from build123d import *

# Parameters (mm, degrees)
F0_R      = 26.5
F1_DEPTH  = 200
F2_R      = 12.5
F3_DEPTH  = 30
F4_W      = 21.5
F4_H      = 60
F5_DEPTH  = 55
F8_DEPTH  = 10
F9_R      = 10
F10_DEPTH = 140


with BuildPart() as f1:
    # F0 (on Front) → F1 (new body)
    with BuildSketch(Plane.XZ):
        Circle(F0_R)
    extrude(amount=F1_DEPTH)

    # F2 (on Right) → F3 (cut, symmetric)
    with BuildSketch(Plane.YZ):
        with Locations((-20, 0)):
            Circle(F2_R)
    extrude(amount=F3_DEPTH, both=True, mode=Mode.SUBTRACT)

    # F4 (on Front) → F5 (cut)
    with BuildSketch(Plane.XZ):
        Rectangle(F4_W, F4_H)
    extrude(amount=F5_DEPTH, mode=Mode.SUBTRACT)

    # F7 (on offset) → F8 (cut)
    with BuildSketch(Plane.YZ.offset(22)):
        with BuildLine():
            Line((-42.6307463948, 4.9999999723), (-172.6307456746, 4.986315794))
            ThreePointArc((-172.6307456746, 4.986315794), (-177.630219249, -0.0147382518), (-172.6286375277, -5.0136839281))
            Line((-172.6286375277, -5.0136839281), (-42.6286382479, -4.9999997498))
            ThreePointArc((-42.6286382479, -4.9999997498), (-37.6302201914, 0.0010540735), (-42.6307463948, 4.9999999723))
        make_face()
    extrude(amount=F8_DEPTH, mode=Mode.SUBTRACT)

    # F9 (on face) → F10 (cut)
    with BuildSketch(Plane.XZ.offset(200)):
        Circle(F9_R)
    extrude(amount=-F10_DEPTH, mode=Mode.SUBTRACT)


solid = f1.part
Design review of the part built by this model. Coordinates are the model's own, in mm. A direction names the side the tool comes from. Give positions to 0.01 mm unless a question says otherwise; leave off trailing zeros. Loops run counter-clockwise (first coordinate to the right, second up) from the corner with the lowest first, then second, coordinate; pieces in that order, holes last. Notation, with made-up numbers: M 20.25,25 L 42.25,25 A15 ccw 42.25,36 Z; hole C -5.5,-23 d9. An arc over 180 degrees is marked long. Answer as a JSON object with one key per item and string values.
Item 1: Wall thickness on line 1 along Y through (x, z) = (14.5, 0); line 2 along Z through (x, y) = (0, -156); line 3 along X through (y, z) = (-151, -7.5): over which ranges is each line inside the solid? List them lowest first.
Output values:
{"line 1": "y = -200 to -32.5, -7.5 to 0", "line 2": "z = -26.5 to -10, 10 to 26.5", "line 3": "x = -25.42 to -6.61, 6.61 to 25.42"}
Item 2: We need section A-A (z = 7). State the section outline as (x, y) points.
Output values:
{"outline": "M -25.56,-200 L -7.14,-200 L -7.14,-60 L 7.14,-60 L 7.14,-200 L 25.56,-200 L 25.56,-30.36 L 10.75,-30.36 L 10.75,-55 L -10.75,-55 L -10.75,-30.36 L -25.56,-30.36 Z; M -25.56,-9.64 L -10.75,-9.64 L -10.75,0 L -25.56,0 Z; M 10.75,-9.64 L 25.56,-9.64 L 25.56,0 L 10.75,0 Z"}
Item 3: We need section C-C (y = -20). State the section outline as (x, z) points.
Output values:
{"outline": "M -23.37,-12.5 A26.5 ccw -10.75,-24.22 L -10.75,-12.5 Z; M -23.37,12.5 L -10.75,12.5 L -10.75,24.22 A26.5 ccw Z; M 10.75,-24.22 A26.5 ccw 23.37,-12.5 L 10.75,-12.5 Z; M 10.75,12.5 L 23.37,12.5 A26.5 ccw 10.75,24.22 Z"}
Item 4: Machinability: for faces 1 (the face through (-2.17, -130.98, -9.76)), 2 (the face through (10.75, -33, 0)), 3 (the face through (24.22, -177.63, 0.1)), 4 (the face through (11, -200, 0)), 5 (the face through (-18.515, -8.077, 3.755)), which of the approach directions +Z, -Z, +X, -X, +Y, -Y give a long, thin tool a straight path to every point of the face, cutting with its end or side? Answer none if there is none.
Output values:
{"face 1": "-Y", "face 2": "+Z, -Z, +Y", "face 3": "+X", "face 4": "+Z, -Z, +X, -X, -Y", "face 5": "+X, -X"}
Item 5: We need section D-D (x = 0). State the section outline as (y, z) points.
Output values:
{"outline": "M -200,-26.5 L -55,-26.5 L -55,26.5 L -200,26.5 L -200,10 L -60,10 L -60,-10 L -200,-10 Z"}
Item 6: For P1, Ø5, axis at y = -108, z = 1, coming from the +X side; P2, Ø1, axis at x = 8, z = 15, coming from the +Y side; P3, Ø20, axis at y = -20, z = 0, coming from the -X side; P4, Ø2, axis at y = -85.5, z = 21, coming from the -X side, all flat-tipped, find the tip position at first contact; note any pin that passes through.
Output values:
{"P1": "stops at x = 22", "P2": "stops at y = -55", "P3": "passes through", "P4": "stops at x = -17.39"}
Item 7: We need section B-B (x = -14). State the section outline as (y, z) points.
Output values:
{"outline": "M -200,-22.5 L 0,-22.5 L 0,22.5 L -200,22.5 Z; hole C -20,0 d25"}
Item 8: Mouldability with a two-part tool opening along Z and no side actions: class faces 6 (the face through (25.276, -98.6, 7.96)), 7 (the face through (22, -109, 0)), 8 (the face through (-10.75, -33, 0)) as pulls with the +Z half, pulls with the -Z half, needs draft (parallel to the pull), parting line crosses it, or undercut.
Output values:
{"face 6": "parting line crosses it", "face 7": "undercut", "face 8": "needs draft"}
